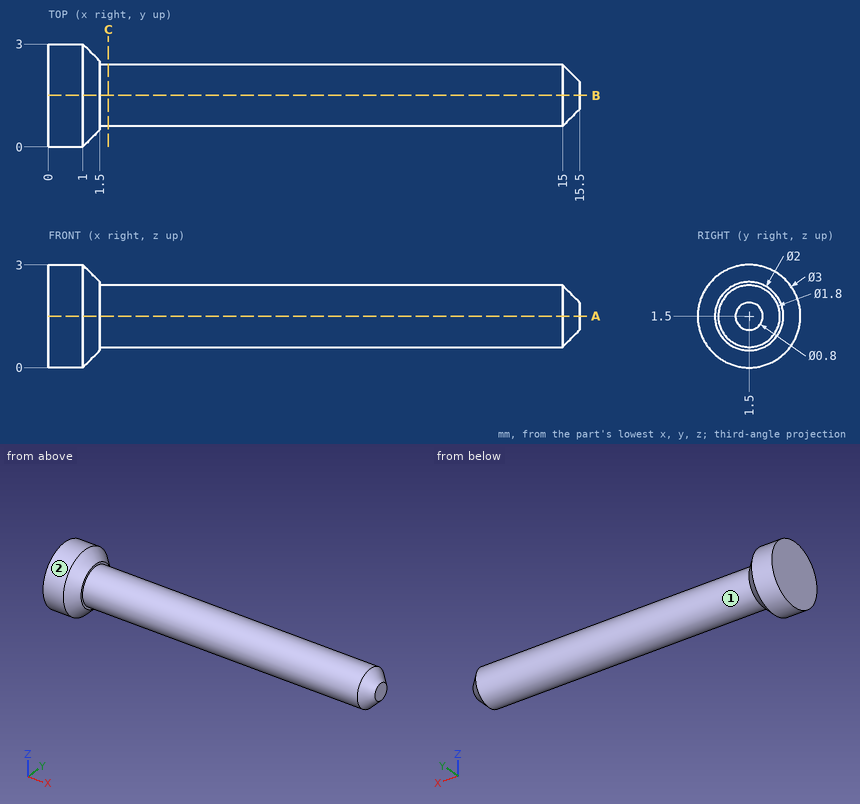
Geometry check sheet. Reference: drawing and pictorial views, mm from the part's lowest x, y, z. A direction names the side the tool comes from. Give positions to 0.01 mm unless a question says otherwise; leave off trailing zeros. Write each loop counter-clockwise with the first axis right and the second up, starting at its lowest first coordinate (ties: lowest second). Pieces come first, ordered by that corner, then holes.
Item 1: Access from +Z, -Z, +X, -X, +Y, -Y to the whole of each face (thin tool, end or side, straight path). Record for the marked faces 1 and 2.
Item 2: Scan lines: L1, parallel to X at y = 1.75, z = 0.7; L2, parallel to Y at x = 11, z = 2.25. Record each from-to range of solid material in increasing order.
Item 3: Gauge pin test, flat end, axial feed: pin 1 (1.5 mm diameter, centred on x = 3, z = 2, fed in from +Y). Record the tip position at first contact, or that the pin passes through.
Item 4: Cross-section at C-C (x = 1.75). Enter the section's corners in (y, z).
Item 5: Cross-section at A-A (z = 1.5). Enter the section's corners in (x, y), and give its area (3 significant figures).
Report:
1. face 1: +X
1. face 2: +X, -X
2. L1: x = 0 to 15.06
2. L2: y = 1 to 2
3. pin 1: stops at y = 2.4
4. outline: circle Ø1.8 at (1.5, 1.5)
5. outline: (0, 0) - (1, 0) - (1.5, 0.5) - (1.5, 0.6) - (15, 0.6) - (15.5, 1.1) - (15.5, 1.9) - (15, 2.4) - (1.5, 2.4) - (1.5, 2.5) - (1, 3) - (0, 3) - close
5. area: 29.2 mm2
